The model under review builds one solid part; all positions refer to its coordinate system, in mm. Round coordinates to 2 decimals unless told otherwise and drop trailing zeros. Write each loop counter-clockwise with the first axis right and the second up, starting at its lowest first coordinate (ties: lowest second). Pieces come first, ordered by that corner, then holes. Notation, with made-up numbers: M 30.5,11.5 L 58.5,11.5 A25 ccw 58.5,31.5 Z; hole C 30.25,-26 d2. An arc over 180 degrees is marked long. One line per item, written item: value. Start each with the question number.
1) Wall thickness on probe 1 along Y at (x, z) = (-2, -9); probe 2 along X at (y, z) = (-0.5, -6.75); probe 3 along Z at (x, y) = (-6, -6.5): over which ranges is each line inside the solid? List them lowest first.
2) Take a section at D-D, the plane y = 8.5. Write out the cut boundary in (x, z), and give its area (3 significant figures).
3) Take a section at A-A, the plane z = -4. Write out the cut boundary in (x, y), and give its area (3 significant figures).
4) For P1, Ø4, axis at x = 1.5, y = -7.5, coming from the +Z side; P2, Ø3, axis at x = 5, y = -1.5, coming from the +Z side; P3, Ø3, axis at x = 7, z = -5, coming from the +Y side, all flat-tipped, find the tip position at first contact; note any pin that passes through.
5) Take a section at C-C, the plane z = 8. Write out the cut boundary in (x, y), and give its area (3 significant figures).
6) Take a section at B-B, the plane y = -3.5. Write out the cut boundary in (x, z), and give its area (3 significant figures).
from build123d import *

# Parameters (mm, degrees)
F0_R     = 10
F1_DEPTH = 38.1
F4_COUNT = 3


with BuildPart() as f1:
    # F0 (on Front) → F1 (new body, symmetric)
    with BuildSketch(Plane.XZ):
        Circle(F0_R)
    extrude(amount=F1_DEPTH, both=True)


with BuildPart() as f4_1:
    # F4: instance of F1
    add(f1.part.rotate(Axis((-10, 10, 10), (-0.5773502692, 0.5773502692, 0.5773502692)), 1 * 360 / F4_COUNT))


with BuildPart() as f4_2:
    # F4: instance of F1
    add(f1.part.rotate(Axis((-10, 10, 10), (-0.5773502692, 0.5773502692, 0.5773502692)), 2 * 360 / F4_COUNT))

    # F5: intersect F4_1, F1
    add(f4_1.part, mode=Mode.INTERSECT)
    add(f1.part, mode=Mode.INTERSECT)


solid = f4_2.part
Checked values:
1. probe 1: y = -4.36 to 4.36
1. probe 2: x = -7.38 to 7.38
1. probe 3: z = -7.6 to 7.6
2. outline: M -5.27,-5.27 L 5.27,-5.27 L 5.27,5.27 L -5.27,5.27 Z
2. area: 111 mm2
3. outline: M -9.17,-4 A10 ccw -4,-9.17 L 4,-9.17 A10 ccw 9.17,-4 L 9.17,4 A10 ccw 4,9.17 L -4,9.17 A10 ccw -9.17,4 Z
3. area: 296 mm2
4. P1: stops at z = 8.35
4. P2: stops at z = 9.37
4. P3: stops at y = 8.35
5. outline: M -6,-6 L 6,-6 L 6,6 L -6,6 Z
5. area: 144 mm2
6. outline: M -9.37,-3.5 A10 ccw -3.5,-9.37 L 3.5,-9.37 A10 ccw 9.37,-3.5 L 9.37,3.5 A10 ccw 3.5,9.37 L -3.5,9.37 A10 ccw -9.37,3.5 Z
6. area: 302 mm2
